The listing builds one solid part. Answer for the finished solid, in the listing's coordinates (mm). Give positions to 0.01 mm unless a question says otherwise; leave off trailing zeros. Order: outer loops, then holes, each group sorted by start corner. A loop starts at its lowest first (then second) coordinate and runs counter-clockwise, first axis right, second up.
```python
from build123d import *

# Parameters (mm, degrees)
R_VOLUTION1_ANGLE       = 180
ESQUISSE2_R             = 9
ENL_V_MAT_EXTRU_1_DEPTH = 36


with BuildPart() as part:
    # Esquisse1 → Révolution1 (revolve)
    with BuildSketch(Plane.XY):
        with BuildLine():
            Line((0, 17), (0, 90))
            Line((0, 90), (2, 90))
            ThreePointArc((2, 90), (17.5, 74.5), (33, 90))
            Line((33, 90), (35, 90))
            Line((35, 90), (35, 17))
            Line((35, 17), (0, 17))
        make_face()
    revolve(axis=Axis((0, 0, 0), (1, 0, 0)), revolution_arc=R_VOLUTION1_ANGLE)

    # Esquisse2 → Enlèv. mat.-Extru.1 (cut, through all)
    with BuildSketch(Plane.ZY):
        with Locations((13, -56.524331044)):
            Circle(ESQUISSE2_R)
        with Locations((58, 0)):
            Circle(ESQUISSE2_R)
        with Locations((13, 56.524331044)):
            Circle(ESQUISSE2_R)
    extrude(amount=-ENL_V_MAT_EXTRU_1_DEPTH, mode=Mode.SUBTRACT)


solid = part.part
```
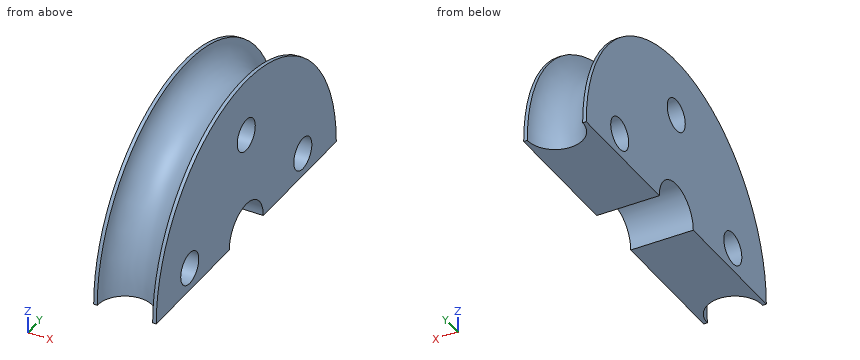
1) Given P1, Ø2, axis at x = 11.5, z = 26.5, coming from the -Y side; P2, Ø1, axis at x = 15, z = 15.5, coming from the -Y side; P3, Ø6, axis at x = 9.5, y = 15, coming from the +Z side, each flat-ended and moving along its own axis, determine where each tip first touches the part or whether it passes through.
Geometry says:
P1: stops at y = -71.53
P2: stops at y = -73.21
P3: stops at z = 77.7
2) Find section A-A (y = 0). Write down the section's boundary in (x, z), then the cut area to 3 significant figures.
Geometry says:
outline: (0, 17) - (35, 17) - (35, 49) - (0, 49) - close; (0, 67) - (35, 67) - (35, 90) - (33, 90) arc R15.5 cw to (2, 90) - (0, 90) - close
area: 1,550 mm2
3) Straight lines are drawn through the part: probe 1 along Y at (x, z) = (11, 13); probe 2 along Y at (x, z) = (27.5, 8); probe 3 along X at (y, z) = (-50, 72.5). For each, find the intervals that lie inside material, in ascending order.
Geometry says:
probe 1: y = -74.81 to -65.52, -47.52 to -10.95, 10.95 to 47.52, 65.52 to 74.81
probe 2: y = -77.75 to -64.01, -49.04 to -15, 15 to 49.04, 64.01 to 77.75
probe 3: x = 0 to 2.12, 32.88 to 35
4) Find section B-B (z = 13). Count the separate pieces of the cut face and the enclosed holes in it, then the cut area to 3 significant figures.
Geometry says:
separate pieces: 4
enclosed holes: 0
area: 3,440 mm2
